Source: CAD feature listing. Evaluate the final solid. Frame: model axes, mm. A direction names the side the tool comes from. Coordinates: 2 decimals unless noted, no trailing zeros. Order: outer loops, then holes, each group sorted by start corner. A loop starts at its lowest first (then second) coordinate and runs counter-clockwise, first axis right, second up.
Item 1: Ray query, line 1 (X direction, y = 5, z = 6.5); line 2 (Z direction, x = 5, y = 0.5); line 3 (Y direction, x = 11.5, z = -9.6). Return the intervals inside material, ascending.
Item 2: Section A-A on x = -5. Return the cut outline in (y, z).
Item 3: Contact query for flat-ended pins moving along their axis: P1, Ø1.5, axis at x = 5, z = -10.5, coming from the -Y side; P2, Ø2.5, axis at y = 0, z = -9.6, coming from the +X side; P3, Ø2.5, axis at x = 5, z = -9.6, coming from the -Y side; P4, Ø4.5, axis at x = 0, z = 6.5, coming from the -Y side. Output: stop coordinate, or through.
Item 4: Mould query, pull axis Z, two halves, no side actions, for faces 1 (the flat face through (0, -9.5, 1)), 2 (the flat face through (0, 0, -38)), 3 (the flat face through (5, 3.5, -10)), 4 (the cylindrical face through (-2.615, -0.133, -8.849)). Classes: released by +Z, released by -Z, zero draft, split by the parting line, or undercut.
Item 5: Reachability of faces 5 (the flat face through (25.5, 0, -1)), 6 (the cylindrical face through (3.57, -3.09, -10.05)) from +Z, -Z, +X, -X, +Y, -Y: full face, straight path, thin tool, end or side. Return the list, or none.
from build123d import *

# Parameters (mm, degrees)
F0_W     = 51
F0_H     = 76
F1_DEPTH = 9.5
F3_DEPTH = 19.001
F2_R     = 2.5
F4_DEPTH = 19.001
F5_DEPTH = 13
F7_DEPTH = 20.5


with BuildPart() as f1:
    # F0 (on Front) → F1 (new body, symmetric)
    with BuildSketch(Plane.XZ):
        Rectangle(F0_W, F0_H)
    extrude(amount=F1_DEPTH, both=True)

    # F2 (on face) → F3 (cut, through all)
    with BuildSketch(Plane.XZ.offset(9.5)):
        with BuildLine():
            ThreePointArc((2.5, 6.5), (-1.767767, 8.267767), (0, 4))
            ThreePointArc((0, 4), (1.767767, 4.732233), (2.5, 6.5))
        make_face()
    extrude(amount=-F3_DEPTH, mode=Mode.SUBTRACT)

    # F2 (on face) → F4 (cut, through all)
    with BuildSketch(Plane.XZ.offset(9.5)):
        with Locations((-5, -9.6)):
            Circle(F2_R)
    extrude(amount=-F4_DEPTH, mode=Mode.SUBTRACT)

    # F2 (on face) → F5 (cut)
    with BuildSketch(Plane.XZ.offset(9.5)):
        with BuildLine():
            ThreePointArc((6.5, -9.6), (5, -8.1), (3.5, -9.6))
            ThreePointArc((3.5, -9.6), (5, -11.1), (6.5, -9.6))
        make_face()
    extrude(amount=-F5_DEPTH, mode=Mode.SUBTRACT)

    # F6 (on face) → F7 (cut)
    with BuildSketch(Plane.YZ.offset(25.5)):
        with BuildLine():
            ThreePointArc((0, -8.1), (-1.06066, -10.66066), (1.5, -9.6))
            ThreePointArc((1.5, -9.6), (1.06066, -8.53934), (0, -8.1))
        make_face()
    extrude(amount=-F7_DEPTH, mode=Mode.SUBTRACT)


solid = f1.part
Answer list:
1. line 1: x = -25.5 to -2.5, 2.5 to 25.5
1. line 2: z = -38 to -11.1, -8.1 to 38
1. line 3: y = -9.5 to -1.5, 1.5 to 9.5
2. outline: (-9.5, -38) - (9.5, -38) - (9.5, -12.1) - (-9.5, -12.1) - close; (-9.5, -7.1) - (9.5, -7.1) - (9.5, 38) - (-9.5, 38) - close
3. P1: stops at y = -9.5
3. P2: stops at x = 4.17
3. P3: stops at y = 3.5
3. P4: passes through
4. face 1: zero draft
4. face 2: released by -Z
4. face 3: undercut
4. face 4: undercut
5. face 5: +Z, -Z, +X, +Y, -Y
5. face 6: -Y
